Input: part model. Units: mm. Frame: model coordinates. Face numbers are marked on the shaded views. A direction names the side the tool comes from. Coordinates: 2 decimals unless noted, no trailing zeros. Write each loop counter-clockwise with the first axis right and the second up, starting at its lowest first coordinate (ties: lowest second). Pieces come first, ordered by that corner, then holes.
1) Section query B-B (z = 4.5). Output: boundary loops of the cut face in (x, y), then the cut area to 3 significant figures.
2) Line query: L1, parallel to X at y = 5.5, z = 3; L2, parallel to Z at x = 5, y = 1.4; L3, parallel to Y at x = 17.75, z = 3.5. Output: solid intervals per line, ascending.
3) Draft query along X for the marked faces 3, 4 and 5. Return one class per face: pulls with the +X half, pulls with the -X half, needs draft (parallel to the pull), parting line crosses it, or undercut.
4) Section query A-A (x = 15). Output: boundary loops of the cut face in (y, z) (3 decimals), then the cut area to 3 significant figures.
5) Section query D-D (x = 5). Output: boundary loops of the cut face in (y, z).
6) Set-up query: the marked faces 1 and 2. Return all of +Z, -Z, +X, -X, +Y, -Y with unobstructed straight access to the full face (end or side cutting, diameter ignored); none if empty.
7) Pin query (flat end, axial travel): pin 1 Ø3.5 at (x, z) = (15, 6) entering from +Y; pin 2 Ø2 at (x, z) = (9.73, 4.1) entering from +Y; pin 3 Ø1.4 at (x, z) = (11, 9) entering from +Y; pin 4 Ø3.5 at (x, z) = (5, 6) entering from -Y. Return the tip coordinate at first contact, or that it passes through.
8) Section query C-C (y = 0.75). Output: boundary loops of the cut face in (x, z) (3 decimals), then the cut area to 3 significant figures.
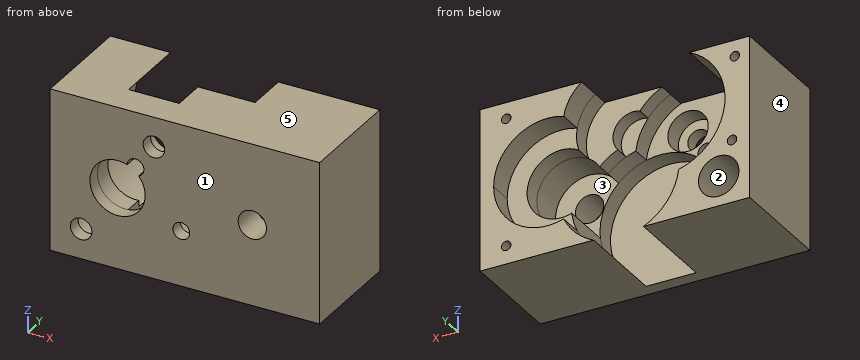
from build123d import *

# Parameters (mm, degrees)
SKETCH_1_W           = 20
SKETCH_1_H           = 12
SKETCH_1_R           = 0.625
SKETCH_1_R_2         = 1.05
EXTRUDE_1_DEPTH      = 1
SKETCH_3_R           = 1.05
EXTRUDE_5_DEPTH      = 1.4
EXTRUDE_START        = 1.4
EXTRUDE_6_DEPTH      = 1.4
EXTRUDE_START_2      = 2.8
EXTRUDE_7_DEPTH      = 1.1
EXTRUDE_START_3      = 3.9
EXTRUDE_8_DEPTH      = 1.3
EXTRUDE_START_4      = 5.2
EXTRUDE_9_DEPTH      = 1.8
SKETCH_5_R           = 0.8
CUT_EXTRUDE_9_DEPTH  = 25.657656012
CUT_EXTRUDE_START    = 8
SKETCH_5_7_R         = 1.5
CUT_EXTRUDE_10_DEPTH = 7
SKETCH_6_R           = 0.35
CUT_EXTRUDE_11_DEPTH = 2


with BuildPart() as part:
    # 草图1 → 凸台-拉伸1 (new body)
    with BuildSketch(Plane(origin=(0, 0, 0), x_dir=(1, 0, 0), z_dir=(0, 1, 0))):
        with Locations((10, -6)):
            Rectangle(SKETCH_1_W, SKETCH_1_H)
        with BuildLine():
            ThreePointArc((5.706865228, -7.92427689), (3.318992309, -4.826665802), (7.05, -6))
            ThreePointArc((7.05, -6), (6.925573765, -6.70332473), (6.567399341, -7.321271852))
            ThreePointArc((6.567399341, -7.321271852), (6.850107647, -7.55134445), (6.956393556, -7.9))
            ThreePointArc((6.956393556, -7.9), (6.343534292, -8.524882071), (5.706865228, -7.92427689))
        make_face(mode=Mode.SUBTRACT)
        with Locations(Location((9.732863826, -4.1, 0), (0, 0, 270))):
            Circle(SKETCH_1_R, mode=Mode.SUBTRACT)
        with Locations(Location((15, -6, 0), (0, 0, 270))):
            Circle(SKETCH_1_R_2, mode=Mode.SUBTRACT)
    extrude(amount=EXTRUDE_1_DEPTH)

    # 草图3 → 凸台-拉伸5 (add)
    with BuildSketch(Plane(origin=(0, 1, 0), x_dir=(1, 0, 0), z_dir=(0, 1, 0))):
        with BuildLine():
            Line((7.878140127, 0), (0, 0))
            Line((0, 0), (0, -12))
            Line((0, -12), (20, -12))
            Line((20, -12), (20, 0))
            Line((20, 0), (11.587587526, 0))
            ThreePointArc((11.587587526, 0), (13.547414344, -6.487300641), (6.856030701, -7.560322408))
            ThreePointArc((6.856030701, -7.560322408), (6.520100415, -8.495831118), (5.706865228, -7.92427689))
            ThreePointArc((5.706865228, -7.92427689), (2.964398818, -6.24254449), (5.234934356, -3.963506482))
            ThreePointArc((5.234934356, -3.963506482), (5.989016009, -1.60328145), (7.878140127, 0))
        make_face()
        with Locations(Location((15, -6, 0), (0, 0, 270))):
            Circle(SKETCH_3_R, mode=Mode.SUBTRACT)
    extrude(amount=EXTRUDE_5_DEPTH)

    # 草图3<11> → 凸台-拉伸6 (add)
    with BuildSketch(Plane(origin=(0, 1, 0), x_dir=(1, 0, 0), z_dir=(0, 1, 0)).offset(EXTRUDE_START)):
        with BuildLine():
            Line((7.878140127, 0), (0, 0))
            Line((0, 0), (0, -12))
            Line((0, -12), (4.476669857, -12))
            ThreePointArc((4.476669857, -12), (1.850964776, -7.48076505), (5.2694824, -3.527089677))
            ThreePointArc((5.2694824, -3.527089677), (6.1148943, -1.424126963), (7.878140127, 0))
        make_face()
        with BuildLine():
            Line((20, 0), (11.587587526, 0))
            ThreePointArc((11.587587526, 0), (13.37352153, -1.455078171), (14.205367203, -3.603297324))
            ThreePointArc((14.205367203, -3.603297324), (17.375189654, -6.856795836), (12.858337915, -7.337500846))
            ThreePointArc((12.858337915, -7.337500846), (11.902158059, -8.042608595), (10.794774983, -8.472910323))
            ThreePointArc((10.794774983, -8.472910323), (9.959364954, -10.562296665), (8.216792734, -11.985984574))
            ThreePointArc((8.216792734, -11.985984574), (8.225940362, -11.993007377), (8.235111081, -12))
            Line((8.235111081, -12), (20, -12))
            Line((20, -12), (20, 0))
        make_face()
    extrude(amount=EXTRUDE_6_DEPTH)

    # 草图3<12> → 凸台-拉伸7 (add)
    with BuildSketch(Plane(origin=(0, 1, 0), x_dir=(1, 0, 0), z_dir=(0, 1, 0)).offset(EXTRUDE_START_2)):
        with BuildLine():
            Line((7.878140127, 0), (0, 0))
            Line((0, 0), (0, -12))
            Line((0, -12), (4.476669857, -12))
            ThreePointArc((4.476669857, -12), (1.850964776, -7.48076505), (5.2694824, -3.527089677))
            ThreePointArc((5.2694824, -3.527089677), (6.1148943, -1.424126963), (7.878140127, 0))
        make_face()
        with BuildLine():
            Line((20, 0), (11.587587526, 0))
            ThreePointArc((11.587587526, 0), (13.37352153, -1.455078171), (14.205367203, -3.603297324))
            ThreePointArc((14.205367203, -3.603297324), (17.375189654, -6.856795836), (12.858337915, -7.337500846))
            ThreePointArc((12.858337915, -7.337500846), (12.228802722, -7.844367641), (11.518753038, -8.230447884))
            ThreePointArc((11.518753038, -8.230447884), (11.618245347, -10.06420032), (9.882502664, -10.663986994))
            ThreePointArc((9.882502664, -10.663986994), (9.128861159, -11.424794322), (8.216792734, -11.985984574))
            ThreePointArc((8.216792734, -11.985984574), (8.225940362, -11.993007377), (8.235111081, -12))
            Line((8.235111081, -12), (20, -12))
            Line((20, -12), (20, 0))
        make_face()
    extrude(amount=EXTRUDE_7_DEPTH)

    # 草图3<13> → 凸台-拉伸8 (add)
    with BuildSketch(Plane(origin=(0, 1, 0), x_dir=(1, 0, 0), z_dir=(0, 1, 0)).offset(EXTRUDE_START_3)):
        with BuildLine():
            Line((7.878140127, 0), (0, 0))
            Line((0, 0), (0, -12))
            Line((0, -12), (4.476669857, -12))
            ThreePointArc((4.476669857, -12), (1.850964776, -7.48076505), (5.2694824, -3.527089677))
            ThreePointArc((5.2694824, -3.527089677), (6.1148943, -1.424126963), (7.878140127, 0))
        make_face()
        with BuildLine():
            Line((20, 0), (11.587587526, 0))
            ThreePointArc((11.587587526, 0), (13.37352153, -1.455078171), (14.205367203, -3.603297324))
            ThreePointArc((14.205367203, -3.603297324), (17.508995457, -6.283842911), (13.690024431, -8.158608118))
            ThreePointArc((13.690024431, -8.158608118), (13.688592195, -10.272489181), (12.470314077, -12))
            Line((12.470314077, -12), (20, -12))
            Line((20, -12), (20, 0))
        make_face()
    extrude(amount=EXTRUDE_8_DEPTH)

    # 草图3<14> → 凸台-拉伸9 (add)
    with BuildSketch(Plane(origin=(0, 1, 0), x_dir=(1, 0, 0), z_dir=(0, 1, 0)).offset(EXTRUDE_START_4)):
        with BuildLine():
            Line((7.878140127, 0), (0, 0))
            Line((0, 0), (0, -12))
            Line((0, -12), (4.476669857, -12))
            ThreePointArc((4.476669857, -12), (1.850964776, -7.48076505), (5.2694824, -3.527089677))
            ThreePointArc((5.2694824, -3.527089677), (6.1148943, -1.424126963), (7.878140127, 0))
        make_face()
        with BuildLine():
            Line((20, 0), (11.587587526, 0))
            ThreePointArc((11.587587526, 0), (12.890484565, -0.893844784), (13.804097772, -2.182956922))
            ThreePointArc((13.804097772, -2.182956922), (17.368162905, -2.776367816), (19, -6))
            ThreePointArc((19, -6), (17.366620176, -9.224764943), (13.80044553, -9.81589689))
            ThreePointArc((13.80044553, -9.81589689), (13.341995684, -11.033778714), (12.470314077, -12))
            Line((12.470314077, -12), (20, -12))
            Line((20, -12), (20, 0))
        make_face()
    extrude(amount=EXTRUDE_9_DEPTH)

    # 草图5 → 切除-拉伸9 (cut, through all)
    with BuildSketch(Plane(origin=(0, 0, 0), x_dir=(1, 0, 0), z_dir=(0, 1, 0))):
        with Locations(Location((2.3, -2.214171161, 0), (0, 0, 270))):
            Circle(SKETCH_5_R)
        with Locations(Location((7.7, -9.785828839, 0), (0, 0, 270))):
            Circle(SKETCH_5_R)
    extrude(amount=CUT_EXTRUDE_9_DEPTH, mode=Mode.SUBTRACT)

    # 草图5<7> → 切除-拉伸10 (cut)
    with BuildSketch(Plane(origin=(0, 0, 0), x_dir=(1, 0, 0), z_dir=(0, 1, 0)).offset(CUT_EXTRUDE_START)):
        with Locations(Location((2.3, -2.214171161, 0), (0, 0, 270))):
            Circle(SKETCH_5_7_R)
        with Locations(Location((7.7, -9.785828839, 0), (0, 0, 270))):
            Circle(SKETCH_5_7_R)
    extrude(amount=-CUT_EXTRUDE_10_DEPTH, mode=Mode.SUBTRACT)

    # 草图6 → 切除-拉伸11 (cut)
    with BuildSketch(Plane(origin=(0, 8, 0), x_dir=(1, 0, 0), z_dir=(0, 1, 0))):
        with Locations(Location((18.067159924, -1.34892989, 0), (0, 0, 270))):
            Circle(SKETCH_6_R)
        with Locations(Location((18.067159924, -10.801482832, 0), (0, 0, 270))):
            Circle(SKETCH_6_R)
        with Locations(Location((1.310630289, -4.626278754, 0), (0, 0, 270))):
            Circle(SKETCH_6_R)
        with Locations(Location((1.101301337, -10.801482832, 0), (0, 0, 270))):
            Circle(SKETCH_6_R)
    extrude(amount=-CUT_EXTRUDE_11_DEPTH, mode=Mode.SUBTRACT)


solid = part.part
Answer:
1. outline: (0, 0) - (3.6, 0) - (3.6, 2.4) - (3.38, 2.4) - (3.38, 8) - (1.64, 8) - (1.64, 6) - (0.98, 6) - (0.98, 8) - (0, 8) - close; (6.4, 0) - (9.25, 0) - (9.25, 1) - (6.4, 1) - close; (10.21, 0) - (20, 0) - (20, 8) - (18.71, 8) - (18.71, 6.2) - (17.03, 6.2) - (17.03, 2.4) - (14.22, 2.4) - (14.22, 1) - (10.21, 1) - close
1. area: 60.6 mm2
2. L1: x = 0 to 1.02, 3.58 to 5.37, 14.1 to 20
2. L2: z = 0 to 3.95, 8.05 to 12
2. L3: y = 0 to 6.2
3. face 3: undercut
3. face 4: pulls with the -X half
3. face 5: needs draft
4. outline: (0, 0) - (8, 0) - (8, 2) - (6.2, 2) - (6.2, 3.475) - (2.4, 3.475) - (2.4, 4.95) - (0, 4.95) - close; (0, 7.05) - (2.4, 7.05) - (2.4, 8.525) - (6.2, 8.525) - (6.2, 10) - (8, 10) - (8, 12) - (0, 12) - close
4. area: 57.4 mm2
5. outline: (0, 0) - (8, 0) - (8, 3.6) - (2.4, 3.6) - (2.4, 3.95) - (0, 3.95) - close; (0, 8.05) - (2.4, 8.05) - (2.4, 12) - (0, 12) - close
6. face 1: +Z, -Z, +X, -X, -Y
6. face 2: +Y
7. pin 1: stops at y = 2.4
7. pin 2: stops at y = 1
7. pin 3: stops at y = 3.8
7. pin 4: passes through
8. outline: (0, 0) - (20, 0) - (20, 12) - (0, 12) - close; hole circle Ø1.6 at (2.3, 2.214); hole (5.707, 7.924) arc R2.05 ccw (long way) to (6.567, 7.321) arc R0.625 ccw (long way) to start; hole circle Ø1.6 at (7.7, 9.786); hole circle Ø1.25 at (9.733, 4.1); hole circle Ø2.1 at (15, 6)
8. area: 217 mm2
